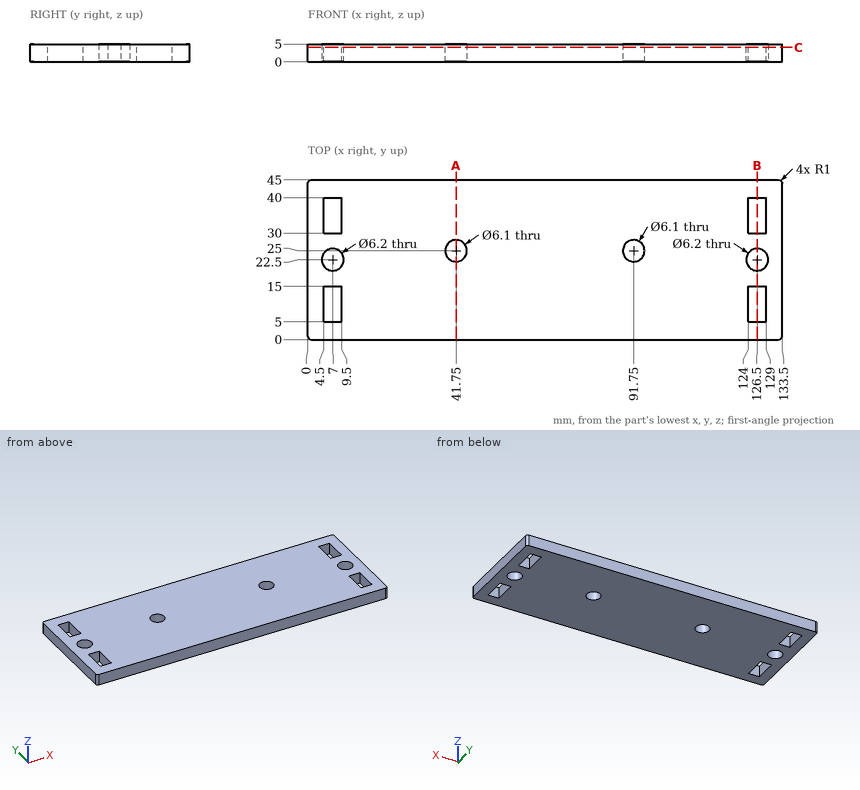
Geometry check sheet. Reference: drawing and pictorial views, mm from the part's lowest x, y, z. Give positions to 0.01 mm unless a question says otherwise; leave off trailing zeros. Order: outer loops, then holes, each group sorted by start corner. A loop starts at its lowest first (then second) coordinate and runs counter-clockwise, first axis right, second up. Notation, with made-up numbers: (-27.5, 46) -> (17.5, 46) arc R30 ccw to (17.5, 73) -> close; hole circle Ø10 at (0.25, 69.25). An arc over 180 degrees is marked (long way). Use CSV: the item, a comma, the result in double quotes. Start each with the question number.
1) Material ranges on line 1 (X direction, y = 33.5, z = 2.5); line 2 (Y direction, x = 7, z = 3.15); line 3 (Y direction, x = 91.75, z = 3.75), recorded low to high. Write a range as from..to.
2) Sectioned sample at B-B, the plane x = 126.5. Record the boundary of the cut face in (y, z).
3) Sectioned sample at A-A, the plane x = 41.75. Record the boundary of the cut face in (y, z).
4) Sectioned sample at C-C, the plane z = 4.05. Give the number of separate pieces and of enclosed holes in the cut face, plus the area to 3 significant figures.
Recorded:
1,line 1,"0..4.5, 9.5..124, 129..133.5"
1,line 2,"0..5, 15..19.4, 25.6..30, 40..45"
1,line 3,"0..21.95, 28.05..45"
2,outline,"(0, 0) -> (5, 0) -> (5, 5) -> (0, 5) -> close; (15, 0) -> (19.4, 0) -> (19.4, 5) -> (15, 5) -> close; (25.6, 0) -> (30, 0) -> (30, 5) -> (25.6, 5) -> close; (40, 0) -> (45, 0) -> (45, 5) -> (40, 5) -> close"
3,outline,"(0, 0) -> (21.95, 0) -> (21.95, 5) -> (0, 5) -> close; (28.05, 0) -> (45, 0) -> (45, 5) -> (28.05, 5) -> close"
4,separate pieces,"1"
4,enclosed holes,"8"
4,area,"5,690 mm2"
